Design review of the part built by this model. Coordinates are the model's own, in mm. Face numbers are marked on the shaded views. Round coordinates to 2 decimals unless told otherwise and drop trailing zeros. Order: outer loops, then holes, each group sorted by start corner. A loop starts at its lowest first (then second) coordinate and runs counter-clockwise, first axis right, second up.
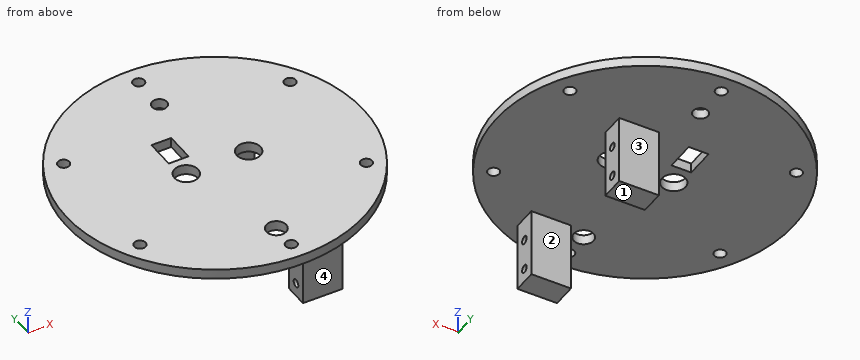
Autodesk Inventor part; units mm, degrees
ref_plane "YZ Plane" through (0, 0, 0) normal (1, 0, 0) x (0, 1, 0)
ref_plane "XZ Plane" through (0, 0, 0) normal (0, 1, 0) x (-1, 0, 0)
ref_plane "XY Plane" through (0, 0, 0) normal (0, 0, 1) x (1, 0, 0)
sketch "Sketch1" plane through (0, 0, 0) normal (0, 0, 1) x (1, 0, 0)
  circle A0 centre (0, 0) radius 47.625
  line L0 (0, 0) -> (0, 41.91)
  line L1 (0, 0) -> (41.91, 0) construction
  circle A1 centre (0, 41.91) radius 1.8415
  circle A2 centre (-36.2951, 20.955) radius 1.8415
  circle A3 centre (-36.2951, -20.955) radius 1.8415
  circle A4 centre (0, -41.91) radius 1.8415
  circle A5 centre (36.2951, -20.955) radius 1.8415
  circle A6 centre (36.2951, 20.955) radius 1.8415
  dimension "d0" = 95.25
  dimension "d1" = 41.91
  dimension "d2" = 90
  dimension "d3" = 3.683
  dimension "d6" = 360
extrude "Extrusion1" add sketch "Sketch1" along normal blind 3.175
sketch "Sketch2" plane through (0, 0, 0) normal (0, 0, -1) x (-1, 0, 0)
  line L0 (-18.415, 17.399) -> (-5.715, 17.399)
  line L1 (-5.715, 17.399) -> (-5.715, 9.779)
  line L2 (-5.715, 9.779) -> (-18.415, 9.779)
  line L3 (-18.415, 9.779) -> (-18.415, 17.399)
  line L4 (-18.415, -30.861) -> (-5.715, -30.861)
  line L5 (-5.715, -30.861) -> (-5.715, -38.481)
  line L6 (-5.715, -38.481) -> (-18.415, -38.481)
  line L7 (-18.415, -38.481) -> (-18.415, -30.861)
  point P0 (0, 0)
  dimension "d10" = 40.64
  dimension "d11" = 9.779
  dimension "d12" = 7.62
  dimension "d13" = 7.62
  dimension "d14" = 12.7
  dimension "d31" = 5.715
extrude "Extrusion2" add sketch "Sketch2" along normal blind 22.225
sketch "Sketch3" plane through (0, 0, 3.175) normal (0, 0, 1) x (1, 0, 0)
  line L0 (-11.1125, 15.875) -> (-4.7625, 15.875)
  line L1 (-4.7625, 15.875) -> (-4.7625, 6.35)
  line L2 (-4.7625, 6.35) -> (-11.1125, 6.35)
  line L3 (-11.1125, 6.35) -> (-11.1125, 15.875)
  point P0 (0, 0)
  dimension "d18" = 6.35
  dimension "d19" = 9.525
  dimension "d33" = 4.7625
  dimension "d34" = 6.35
extrude "Extrusion3" cut sketch "Sketch3" against normal blind 19.05
sketch "Sketch4" plane through (5.715, -38.481, 0) normal (-1, 0, 0) x (0, 0, 1)
  line L0 (0, 7.62) -> (0, 0)
  line L1 (0, 7.62) -> (-22.225, 7.62)
  line L2 (-22.225, 0) -> (-22.225, 7.62)
  line L3 (0, 0) -> (-22.225, 0)
  circle A0 centre (-17.78, 3.81) radius 1.27
  circle A1 centre (-7.62, 3.81) radius 1.27
  line L4 (0, 7.62) -> (-22.225, 7.62)
  line L5 (0, 55.88) -> (0, 48.26)
  line L6 (0, 55.88) -> (-22.225, 55.88)
  line L7 (-22.225, 48.26) -> (-22.225, 55.88)
  line L8 (0, 48.26) -> (-22.225, 48.26)
  circle A2 centre (-17.78, 52.07) radius 1.27
  circle A3 centre (-7.62, 52.07) radius 1.27
  point P0 (0, 38.481)
  dimension "d22" = 2.54
  dimension "d23" = 2.54
  dimension "d24" = 3.81
  dimension "d25" = 10.16
  dimension "d27" = 2.54
  dimension "d28" = 2.54
  dimension "d32" = 4.445
extrude "Extrusion4" cut sketch "Sketch4" against normal blind 19.05 contours A0 | A1 | A2 | A3
sketch "Sketch8" plane through (0, 0, 0) normal (0, 0, -1) x (-1, 0, 0)
  line L0 (11.1125, 15.875) -> (11.1125, 6.35)
  line L1 (11.1125, 6.35) -> (4.7625, 6.35)
  line L2 (4.7625, 6.35) -> (4.7625, 15.875)
  line L3 (4.7625, 15.875) -> (11.1125, 15.875)
  line L4 (-5.715, 17.399) -> (-5.715, 9.779)
  line L5 (-5.715, 9.779) -> (-18.415, 9.779)
  line L6 (-18.415, 9.779) -> (-18.415, 17.399)
  line L7 (-18.415, 17.399) -> (-5.715, 17.399)
  line L8 (-5.715, -30.861) -> (-5.715, -38.481)
  line L9 (-5.715, -38.481) -> (-18.415, -38.481)
  line L10 (-18.415, -38.481) -> (-18.415, -30.861)
  line L11 (-18.415, -30.861) -> (-5.715, -30.861)
  circle A0 centre (-36.2951, 20.955) radius 1.8415
  circle A1 centre (-36.2951, -20.955) radius 1.8415
  circle A2 centre (0, -41.91) radius 1.8415
  circle A3 centre (36.2951, -20.955) radius 1.8415
  circle A4 centre (36.2951, 20.955) radius 1.8415
  circle A5 centre (0, 41.91) radius 1.8415
  circle A6 centre (0, 0) radius 47.625
  circle A7 centre (9.2075, 0) radius 3.81
  circle A8 centre (-10.7925, 0) radius 3.81
  dimension "d42" = 7.62
  dimension "d43" = 6.35
  dimension "d44" = 1.905
  dimension "d45" = 7.62
  dimension "d46" = 20
extrude "Extrusion6" cut sketch "Sketch8" against normal blind 25.4 contours A7 | A8
sketch "Sketch10" plane through (0, 0, 3.175) normal (0, 0, 1) x (1, 0, 0)
  circle A0 centre (0, 30.48) radius 2.3813
  point P0 (0, 0)
  dimension "d53" = 4.7625
  dimension "d54" = 30.48
extrude "Extrusion8" cut sketch "Sketch10" against normal through all
sketch "Sketch11" plane through (0, 0, 0) normal (0, 0, -1) x (-1, 0, 0)
  circle A0 centre (0, -33.655) radius 3.175
  point P0 (0, 0)
  dimension "d57" = 6.35
  dimension "d58" = 33.655
extrude "Extrusion9" cut sketch "Sketch11" against normal blind 25.4
sketch "Sketch9" plane through (0, 0, 3.175) normal (0, 0, 1) x (1, 0, 0)
  circle A0 centre (0, 0) radius 47.625
  circle A1 centre (0, 0) radius 47.625
  circle A2 centre (0, 0) radius 47.117
  dimension "d49" = 95.25
  dimension "d50" = 94.234
extrude "PRINT_FEATURE_1" [suppressed]
properties part number "foreElectronicsSealingWallRear" material "ABS Plastic"
1) Take a section at B-B on x = 0. Give the boundary of the cut face in (y, z) (1 decimal), plus the area to 3 significant figures.
Results:
outline: (-47.6, 0) - (-43.8, 0) - (-43.8, 3.2) - (-47.6, 3.2) - close; (-40.1, 0) - (-36.8, 0) - (-36.8, 3.2) - (-40.1, 3.2) - close; (-30.5, 0) - (28.1, 0) - (28.1, 3.2) - (-30.5, 3.2) - close; (32.9, 0) - (40.1, 0) - (40.1, 3.2) - (32.9, 3.2) - close; (43.8, 0) - (47.6, 0) - (47.6, 3.2) - (43.8, 3.2) - close
area: 244 mm2
2) Take a section at D-D on z = -14.25. Give the boundary of the cut face in (x, y) (3 decimals), plus the area to 3 significant figures.
Results:
outline: (5.715, -38.481) - (18.415, -38.481) - (18.415, -30.861) - (5.715, -30.861) - close; (5.715, 9.779) - (18.415, 9.779) - (18.415, 17.399) - (5.715, 17.399) - close
area: 194 mm2
3) The part is to be moulded in two halves that separate along Y. For the marked faces 1, 2, 3 and 4, say which applies: released by +Y, released by -Y, zero draft, split by the parting line, or undercut.
Results:
face 1: zero draft
face 2: undercut
face 3: released by +Y
face 4: released by -Y
4) Take a section at A-A on z = -7.62. Give the boundary of the cut face in (x, y) (3 decimals).
Results:
outline: (5.715, -38.481) - (18.415, -38.481) - (18.415, -35.941) - (5.715, -35.941) - close; (5.715, -33.401) - (18.415, -33.401) - (18.415, -30.861) - (5.715, -30.861) - close; (5.715, 9.779) - (18.415, 9.779) - (18.415, 12.319) - (5.715, 12.319) - close; (5.715, 14.859) - (18.415, 14.859) - (18.415, 17.399) - (5.715, 17.399) - close
5) Take a section at C-C on y = 0. Give the boundary of the cut face in (x, z) (1 decimal).
Results:
outline: (-47.6, 0) - (-13, 0) - (-13, 3.2) - (-47.6, 3.2) - close; (-5.4, 0) - (7, 0) - (7, 3.2) - (-5.4, 3.2) - close; (14.6, 0) - (47.6, 0) - (47.6, 3.2) - (14.6, 3.2) - close
6) Clearance check with flat-ended pins moving along their axes: P1, Ø3, axis at y = -34.671, z = -17.78, coming from the +X side (3 decimals); P2, Ø10, axis at y = 9, z = -15, coming from the -X side (3 decimals); P3, Ø4, axis at x = 10, z = -8.5, coming from the +Y side. State where each tip first meets the part, or that it passes through.
Results:
P1: stops at x = 18.415
P2: stops at x = 5.715
P3: stops at y = 17.4
7) To check wall thickness, follow line 1 along Y through (x, z) = (15, -17.78); line 2 along Y through (x, z) = (0, 2.55) (1 decimal); line 3 along Z through (x, y) = (7.5, 14.5) (3 decimals). State the ranges of each line that lie inside material, in increasing order.
Results:
line 1: y = -38.48 to -35.94, -33.4 to -30.86, 9.78 to 12.32, 14.86 to 17.4
line 2: y = -47.6 to -43.8, -40.1 to -36.8, -30.5 to 28.1, 32.9 to 40.1, 43.8 to 47.6
line 3: z = -22.225 to -18.665, -16.895 to -8.505, -6.735 to 3.175
